For this review, take the finished solid that the model builds, in its own axes (mm). A direction names the side the tool comes from. Give positions to 0.01 mm unless a question says otherwise; leave off trailing zeros. Order: outer loops, then holes, each group sorted by start corner. A loop starts at its lowest first (then second) coordinate and runs counter-clockwise, first axis right, second up.
Autodesk Inventor part; units mm, degrees
ref_plane "YZ Plane" through (0, 0, 0) normal (1, 0, 0) x (0, 1, 0)
ref_plane "XZ Plane" through (0, 0, 0) normal (0, 1, 0) x (-1, 0, 0)
ref_plane "XY Plane" through (0, 0, 0) normal (0, 0, 1) x (1, 0, 0)
sketch "Эскиз1" plane through (0, 0, 0) normal (0, 0, 1) x (1, 0, 0)
  line L0 (0, 0) -> (21.2967, 0)
  line L1 (0, 0) -> (0, 6)
  line L2 (0, 6) -> (14.75, 6)
  line L3 (14.75, 6) -> (14.75, 5)
  line L4 (14.75, 5) -> (15.75, 5)
  line L5 (15.75, 5) -> (15.75, 14.5)
  line L6 (15.75, 14.5) -> (20.75, 14.5)
  line L7 (20.75, 14.5) -> (20.75, 0)
  dimension "d0" = 12
  dimension "d1" = 10
  dimension "d2" = 29
  dimension "d3" = 1
  dimension "d4" = 14.75
  dimension "d5" = 5
revolve "Вращение1" add sketch "Эскиз1" angle 360 about axis through (0, 0, 0) along (1, 0, 0)
chamfer "Фаска1" distance 1 angle 45 1 edges at (0, -6, 0)
fillet "Сопряжение1" radius 0.5 2 edges at (15.75, -14.5, 0) (20.75, -14.5, 0)
sketch "Эскиз2" plane through (20.75, 0, 0) normal (1, 0, 0) x (0, 0, -1)
  line L0 (5.4848, 9.5) -> (10.9697, 0)
  line L1 (10.9697, 0) -> (5.4848, -9.5)
  line L2 (5.4848, -9.5) -> (-5.4848, -9.5)
  line L3 (-5.4848, -9.5) -> (-10.9697, 0)
  line L4 (-10.9697, 0) -> (-5.4848, 9.5)
  line L5 (-5.4848, 9.5) -> (5.4848, 9.5)
  point P0 (0, 0)
  point P1 (0, 0)
  dimension "d11" = 19
extrude "Выдавливание1" add sketch "Эскиз2" along normal blind 6
sketch "Эскиз3" plane through (0, 0, 0) normal (0, 1, 0) x (-1, 0, 0)
  line L0 (-20.75, 10.9697) -> (-26.75, 10.9697)
  line L1 (-25.3358, 10.9697) -> (-26.75, 9.5554)
  line L2 (-26.75, 5.4848) -> (-26.75, 10.9697)
  line L3 (3.6, 0) -> (-21.6, 0)
  point P0 (0, 0)
  dimension "d14" = 2
  dimension "d15" = 45
revolve "Вращение2" cut sketch "Эскиз3" angle 360 about axis through (-10, 0, 0) along (1, 0, 0)
thread "Резьба1"
properties part number "Слив_масла"
1) We need section A-A on x = 22.5. Give the boundary of the cut face in (y, z), then the cut area to 3 significant figures.
Answer sheet:
outline: (-9.5, -5.48) - (0, -10.97) - (9.5, -5.48) - (9.5, 5.48) - (0, 10.97) - (-9.5, 5.48) - close
area: 313 mm2
2) Clearance check with flat-ended pins moving along their axes: pin 1 (3 mm diameter, centred on x = 15.5, y = -3, fed in from +Z); pin 2 (3 mm diameter, centred on x = 25, z = 2.5, fed in from -Y); pin 3 (2 mm diameter, centred on x = 15, y = -8, fed in from +Z); pin 4 (8 mm diameter, centred on x = 7, z = -10.5, fed in from -Y). State where each tip first meets the part, or that it passes through.
Answer sheet:
pin 1: stops at z = 14.4
pin 2: stops at y = -9.5
pin 3: stops at z = 12.2
pin 4: passes through
3) We need section B-B on z = 0. Give the boundary of the cut face in (x, y).
Answer sheet:
outline: (0, -5) - (1, -6) - (14.75, -6) - (14.75, -5) - (15.75, -5) - (15.75, -14) arc R0.5 ccw to (16.25, -14.5) - (20.25, -14.5) arc R0.5 ccw to (20.75, -14) - (20.75, -9.5) - (26.75, -9.5) - (26.75, 9.5) - (20.75, 9.5) - (20.75, 14) arc R0.5 ccw to (20.25, 14.5) - (16.25, 14.5) arc R0.5 ccw to (15.75, 14) - (15.75, 5) - (14.75, 5) - (14.75, 6) - (1, 6) - (0, 5) - close
4) To check wall thickness, follow line 1 (Y direction, x = 22.25, z = -1.5); line 2 (X direction, y = -1.75, z = 6.25); line 3 (X direction, y = 10, z = -2.75). State the ranges of each line that lie inside material, in increasing order.
Answer sheet:
line 1: y = -9.5 to 9.5
line 2: x = 15.75 to 26.75
line 3: x = 15.75 to 20.75
5) Tool access review of faces 1 (the face through (15.26, -1.08, -4.88)), 2 (the face through (23.708, 4.683, 8.266)), 3 (the face through (20.75, -10, 0)), 4 (the face through (23.7, 4.8, -8.2)): name each direction out of +Z, -Z, +X, -X, +Y, -Y from which nothing blocks a thin tool from reaching the whole face with its end or side.
Answer sheet:
face 1: none
face 2: +Z, +X, +Y
face 3: +X
face 4: -Z, +X, +Y
6) We need section C-C on x = 2. Give the boundary of the cut face in (y, z).
Answer sheet:
outline: circle Ø12 at (0, 0)
